Geometry check sheet. Reference: the model listing, model coordinates, mm. A direction names the side the tool comes from. Round coordinates to 2 decimals unless told otherwise and drop trailing zeros. Write each loop counter-clockwise with the first axis right and the second up, starting at its lowest first coordinate (ties: lowest second). Pieces come first, ordered by that corner, then holes. Notation, with made-up numbers: (80.5, 35.25) - (90.5, 35.25) arc R32 ccw to (90.5, 70.25) - close; hole circle Ø5 at (-5.75, -2). An arc over 180 degrees is marked (long way). Return JSON: item names as keys, results as strings. Group by question number.
from build123d import *

# Parameters (mm, degrees)
BOSS_EXTRUDE1_DEPTH  = 60
CHAMFER1_SIZE        = 5
CHAMFER1_EDGE_2_SIZE = 5
CHAMFER1_EDGE_3_SIZE = 5
SKETCH2_W            = 7
SKETCH2_H            = 4.5
CUT_EXTRUDE1_DEPTH   = 19.5
SKETCH3_R            = 2.2
CUT_EXTRUDE2_DEPTH   = 2.5
CIRPATTERN1_COUNT    = 3


with BuildPart() as part:
    # Sketch1 → Boss-Extrude1 (new body)
    with BuildSketch(Plane.XY):
        Polygon((-20, -11.547005384), (20, -11.547005384), (0, 23.094010768), align=None)
    extrude(amount=BOSS_EXTRUDE1_DEPTH)

    # Chamfer1
    chamfer1_edges = [part.edges().sort_by_distance(p)[0] for p in [
        (0, 23.094010768, 30),
    ]]
    chamfer(chamfer1_edges, length=CHAMFER1_SIZE)

    # Chamfer1 edge 2
    chamfer1_edge_2_edges = [part.edges().sort_by_distance(p)[0] for p in [
        (20, -11.547005384, 30),
    ]]
    chamfer(chamfer1_edge_2_edges, length=CHAMFER1_EDGE_2_SIZE)

    # Chamfer1 edge 3
    chamfer1_edge_3_edges = [part.edges().sort_by_distance(p)[0] for p in [
        (-20, -11.547005384, 30),
    ]]
    chamfer(chamfer1_edge_3_edges, length=CHAMFER1_EDGE_3_SIZE)

    # Sketch2 → Cut-Extrude1 (cut)
    with BuildSketch(Plane.XY.offset(60)):
        with Locations((-10.726497308, -6.797005384)):
            Rectangle(SKETCH2_W, SKETCH2_H)
    cut_extrude1 = extrude(amount=-CUT_EXTRUDE1_DEPTH, mode=Mode.SUBTRACT)

    # Sketch3 → Cut-Extrude2 (cut)
    with BuildSketch(Plane.XZ.offset(11.547005384)):
        with Locations((-10.726497308, 45.5)):
            Circle(SKETCH3_R)
    cut_extrude2 = extrude(amount=-CUT_EXTRUDE2_DEPTH, mode=Mode.SUBTRACT)

    # CirPattern1: Cut-Extrude1, Cut-Extrude2 ×3 about axis
    cirpattern1_axis = Axis((0, 0, 0), (0, 0, 1))
    for i in range(1, CIRPATTERN1_COUNT):
        add(cut_extrude1.rotate(cirpattern1_axis, i * 360 / CIRPATTERN1_COUNT), mode=Mode.SUBTRACT)
        add(cut_extrude2.rotate(cirpattern1_axis, i * 360 / CIRPATTERN1_COUNT), mode=Mode.SUBTRACT)


solid = part.part
1. Material ranges on line 1 along X through (y, z) = (-9, 45); line 2 along Y through (x, z) = (9.5, 48); line 3 along Y through (x, z) = (3, 46), recorded low to high.
2. Section check D-D (y = 5.5). Enter the section's corners in (x, z), and give its area (3 significant figures).
3. Tool access check on faces 4 (the face through (0, -11.547, 30)), 5 (the face through (-14.226, -7, 50)). Record the directions out of +Z, -Z, +X, -X, +Y, -Y that give a thin tool (end or side, any length) a straight path to the whole face; none if there is none.
4. Section check C-C (x = 1). Enter the section's corners in (y, z), and give its area (3 significant figures).
5. Depth check by flat-ended pin: pin 1 Ø2 at (x, z) = (-12, 54) entering from +Y; pin 2 Ø5 at (x, z) = (-12.5, 25.5) entering from +Y; pin 3 Ø2 at (x, y) = (10.5, -4) entering from +Z. Enter the tip coordinate at first touch or a pass-through.
6. Section check A-A (z = 54). Enter the section's corners in (x, y).
7. Mould release check, pull along Z, two halves, no side actions. Record for faces 1 (the face through (1.2, 15.735, 50.386)), 2 (the face through (-9.71, -10.31, 43.55)), 3 (the face through (0, 0, 0)): pulls with the +Z half, pulls with the -Z half, needs draft (parallel to the pull), parting line crosses it, or undercut.
Result sheet:
{
 "1": {"line 1": "x = -16.47 to -14.23, -7.23 to 10.45, 12.86 to 16.47", "line 2": "y = -11.55 to -7.36, -2.86 to 6.64", "line 3": "y = -11.55 to 14.29, 14.7 to 17.9"},
 "2": {"outline": "(-10.16, 0) - (10.16, 0) - (10.16, 60) - (-10.16, 60) - close", "area": "1,220 mm²"},
 "3": {"face 4": "+Z, -Z, +X, -X, -Y", "face 5": "+Z"},
 "4": {"outline": "(-11.55, 0) - (18.76, 0) - (18.76, 60) - (15.85, 60) - (15.85, 40.5) - (10.83, 40.5) - (10.83, 60) - (-11.55, 60) - close", "area": "1,720 mm²"},
 "5": {"pin 1": "stops at y = 4.04", "pin 2": "stops at y = 5.77", "pin 3": "stops at z = 40.5"},
 "6": {"outline": "(-17.5, -7.22) - (-15, -11.55) - (15, -11.55) - (17.5, -7.22) - (2.5, 18.76) - (-2.5, 18.76) - close; hole (-14.23, -9.05) - (-7.23, -9.05) - (-7.23, -4.55) - (-14.23, -4.55) - close; hole (-4.22, 10.78) - (-0.32, 8.53) - (3.18, 14.59) - (-0.72, 16.84) - close; hole (7.55, -3.98) - (11.05, -10.05) - (14.95, -7.8) - (11.45, -1.73) - close"},
 "7": {"face 1": "needs draft", "face 2": "undercut", "face 3": "pulls with the -Z half"}
}
